Verification items for this drawing (mm, ordinates from the low corner). A direction names the side the tool comes from. Coordinates: 2 decimals unless noted, no trailing zeros. Order: outer loops, then holes, each group sorted by start corner. A loop starts at its lowest first (then second) coordinate and runs counter-clockwise, first axis right, second up.
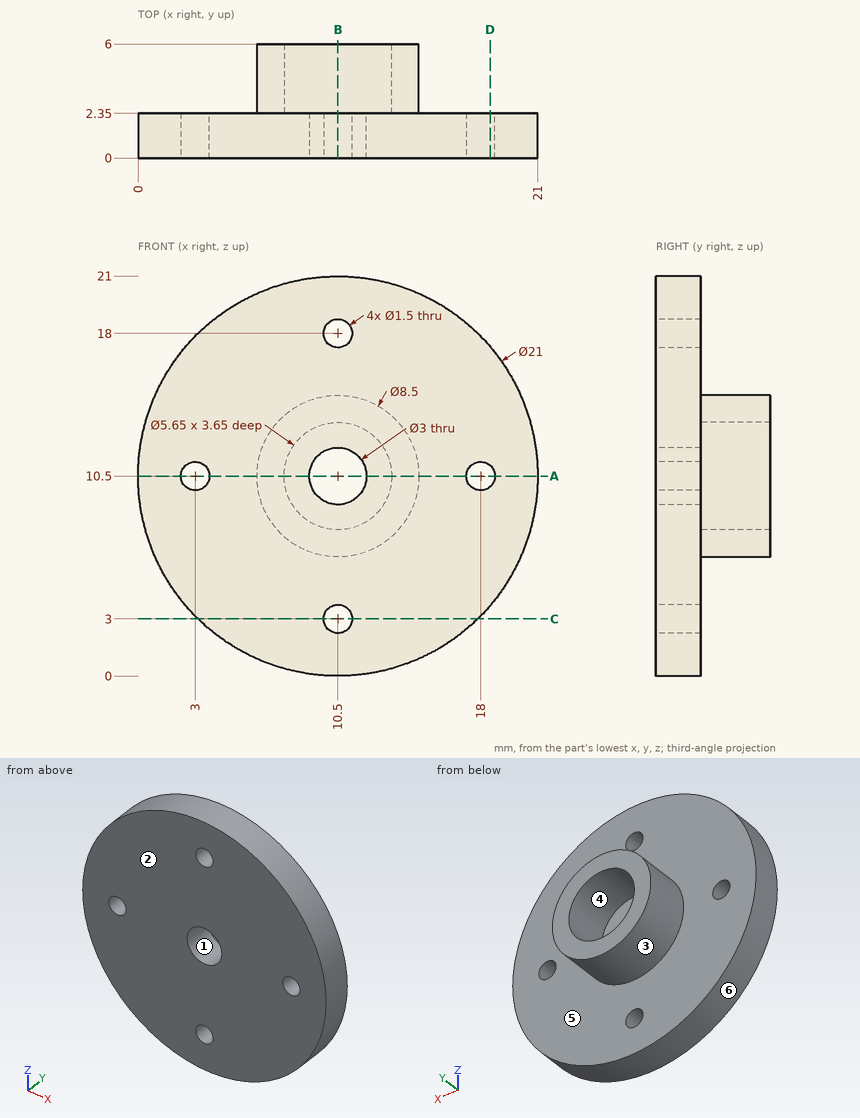
Item 1: Release check for a two-part mould opening along Z. For the marked faces 1, 2, 3 and 4 record: pulls with the +Z half, pulls with the -Z half, needs draft (parallel to the pull), parting line crosses it, or undercut.
Item 2: Sectioned sample at C-C (z = 3). Record the cut outline in (x, y).
Item 3: Sectioned sample at B-B (x = 10.5). Record the cut outline in (y, z) (3 decimals).
Item 4: Thickness scan on line 1 along Z through (x, y) = (10.5, 0.5); line 2 along Y through (x, z) = (17.75, 6.25). Record the ranges inside material, lowest first.
Item 5: Depth check by flat-ended pin: P1, Ø3, axis at x = 10, z = 9.5, coming from the +Y side; P2, Ø2, axis at y = 1.5, z = 4, coming from the -X side. Enter the tip coordinate at first touch or a pass-through.
Item 6: Tool access check on the marked faces 5 and 6. Record the directions out of +Z, -Z, +X, -X, +Y, -Y that give a thin tool (end or side, any length) a straight path to the whole face; none if there is none.
Item 7: Sectioned sample at D-D (x = 18.5). Record the cut outline in (y, z).
Item 8: Sectioned sample at A-A (z = 10.5). Record the cut outline in (x, y) (3 decimals), and give its area (3 significant figures).
Geometry check:
1. face 1: undercut
1. face 2: needs draft
1. face 3: parting line crosses it
1. face 4: undercut
2. outline: (3.15, 0) - (9.75, 0) - (9.75, 2.35) - (3.15, 2.35) - close; (11.25, 0) - (17.85, 0) - (17.85, 2.35) - (11.25, 2.35) - close
3. outline: (0, 0) - (2.35, 0) - (2.35, 2.25) - (0, 2.25) - close; (0, 3.75) - (2.35, 3.75) - (2.35, 6.25) - (6, 6.25) - (6, 7.675) - (2.35, 7.675) - (2.35, 9) - (0, 9) - close; (0, 12) - (2.35, 12) - (2.35, 13.325) - (6, 13.325) - (6, 14.75) - (2.35, 14.75) - (2.35, 17.25) - (0, 17.25) - close; (0, 18.75) - (2.35, 18.75) - (2.35, 21) - (0, 21) - close
4. line 1: z = 0 to 2.25, 3.75 to 9, 12 to 17.25, 18.75 to 21
4. line 2: y = 0 to 2.35
5. P1: stops at y = 2.35
5. P2: stops at x = 1.56
6. face 5: +Y
6. face 6: +Y, -Y
7. outline: (0, 3.7) - (2.35, 3.7) - (2.35, 9.94) - (0, 9.94) - close; (0, 11.06) - (2.35, 11.06) - (2.35, 17.3) - (0, 17.3) - close
8. outline: (0, 0) - (2.25, 0) - (2.25, 2.35) - (0, 2.35) - close; (3.75, 0) - (9, 0) - (9, 2.35) - (7.675, 2.35) - (7.675, 6) - (6.25, 6) - (6.25, 2.35) - (3.75, 2.35) - close; (12, 0) - (17.25, 0) - (17.25, 2.35) - (14.75, 2.35) - (14.75, 6) - (13.325, 6) - (13.325, 2.35) - (12, 2.35) - close; (18.75, 0) - (21, 0) - (21, 2.35) - (18.75, 2.35) - close
8. area: 45.7 mm2
